Source: three-view drawing plus pictorial views. Frame: mm from the lowest corner of the part. Coordinates: 2 decimals unless noted, no trailing zeros. Write each loop counter-clockwise with the first axis right and the second up, starting at its lowest first coordinate (ties: lowest second). Pieces come first, ordered by that corner, then holes. Notation, with made-up numbers: (13, -35.75) -> (70, -35.75) arc R16 cw to (70, -10.75) -> close; hole circle Ø3 at (33, 22). An arc over 180 degrees is marked (long way). One line per item, written item: value.
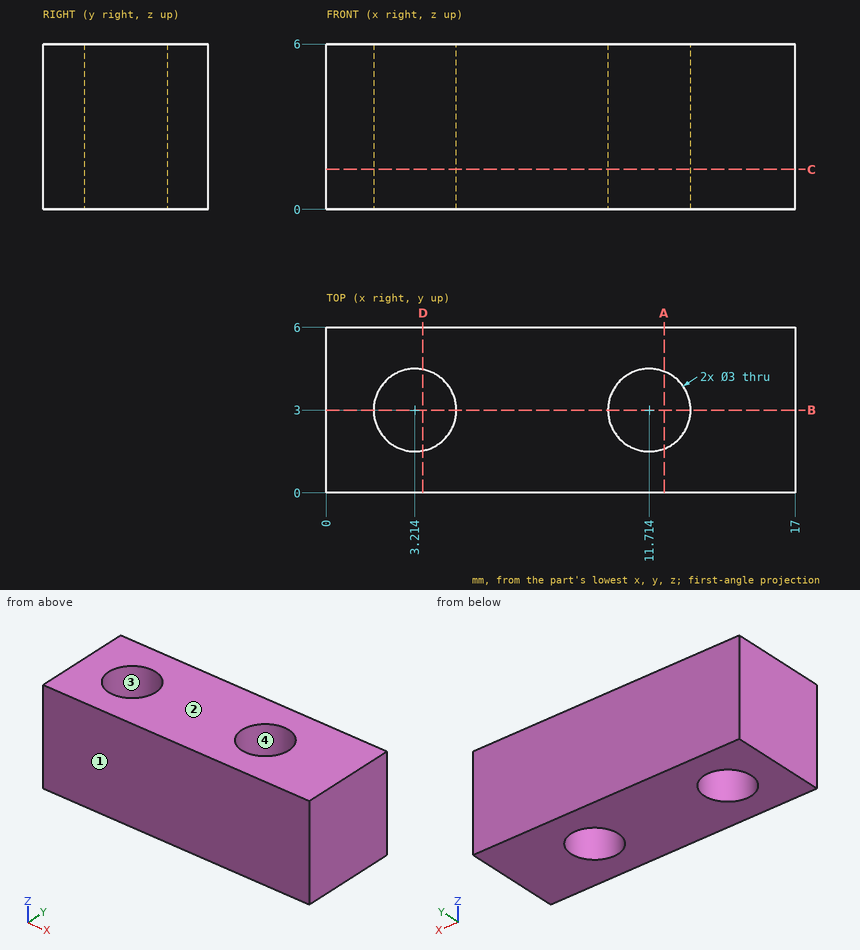
(1) Section D-D (x = 3.5). Return the cut outline in (y, z), then the cut area to 3 significant figures.
Responses:
outline: (0, 0) -> (1.53, 0) -> (1.53, 6) -> (0, 6) -> close; (4.47, 0) -> (6, 0) -> (6, 6) -> (4.47, 6) -> close
area: 18.3 mm2
(2) Line query: line 1 (X direction, y = 3.1, z = 1.75); line 2 (Y direction, x = 4, z = 2.55); line 3 (Y direction, x = 4.5, z = 3.5). Output: solid intervals per line, ascending. Write a range as [from, to].
Responses:
line 1: x = [0, 1.72], [4.71, 10.22], [13.21, 17]
line 2: y = [0, 1.72], [4.28, 6]
line 3: y = [0, 2.23], [3.77, 6]
(3) Section A-A (x = 12.25). Return the cut outline in (y, z), then the cut area to 3 significant figures.
Responses:
outline: (0, 0) -> (1.6, 0) -> (1.6, 6) -> (0, 6) -> close; (4.4, 0) -> (6, 0) -> (6, 6) -> (4.4, 6) -> close
area: 19.2 mm2
(4) Pull-direction query (Y, two-part tool) for the marked faces 1, 2, 3 and 4; classes: released by +Y, released by -Y, zero draft, split by the parting line, or undercut.
Responses:
face 1: released by -Y
face 2: zero draft
face 3: undercut
face 4: undercut
(5) Section C-C (z = 1.45). Return the cut outline in (x, y).
Responses:
outline: (0, 0) -> (17, 0) -> (17, 6) -> (0, 6) -> close; hole circle Ø3 at (3.21, 3); hole circle Ø3 at (11.71, 3)
(6) Section B-B (y = 3). Return the cut outline in (x, z), then the cut area to 3 significant figures.
Responses:
outline: (0, 0) -> (1.71, 0) -> (1.71, 6) -> (0, 6) -> close; (4.71, 0) -> (10.21, 0) -> (10.21, 6) -> (4.71, 6) -> close; (13.21, 0) -> (17, 0) -> (17, 6) -> (13.21, 6) -> close
area: 66.0 mm2
